Work out the finished part from the listing and answer in its coordinate system (mm). Face numbers are marked on the shaded views. A direction names the side the tool comes from. Round coordinates to 2 decimals unless told otherwise and drop trailing zeros. Order: outer loops, then holes, each group sorted by start corner. A loop starts at its lowest first (then second) coordinate and runs counter-clockwise, first axis right, second up. Notation, with made-up numbers: (37, -21.5) -> (85, -21.5) arc R21 cw to (85, 12.5) -> close; hole circle Ø9 at (69, 63.5). An arc over 180 degrees is marked (long way). Use one line per item in the form item = value.
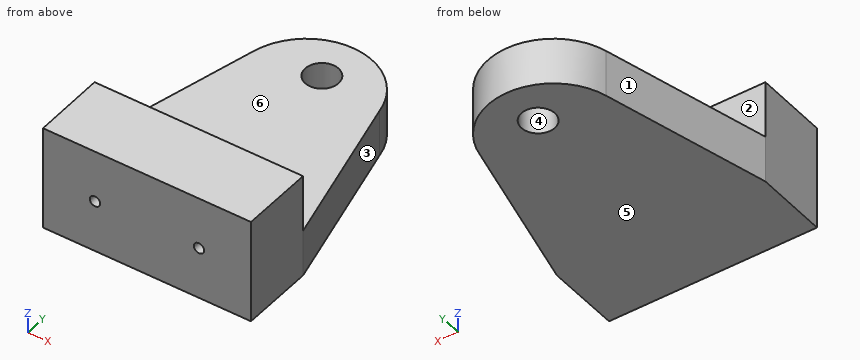
Autodesk Inventor part; units mm, degrees
ref_plane "YZ Plane" through (0, 0, 0) normal (1, 0, 0) x (0, 1, 0)
ref_plane "XZ Plane" through (0, 0, 0) normal (0, 1, 0) x (-1, 0, 0)
ref_plane "XY Plane" through (0, 0, 0) normal (0, 0, 1) x (1, 0, 0)
sketch "Sketch1" plane through (0, 0, 0) normal (0, 0, 1) x (1, 0, 0)
  circle A0 centre (10, 23.5) radius 1.6
  line L0 (-0.0511, 6.9998) -> (3.884, 22.9404)
  line L1 (20, 6.9998) -> (16.1838, 22.6325)
  arc A1 (16.1838, 22.6325) -> (3.884, 22.9404) centre (10, 21.4305) ccw
  line L2 (0, 0) -> (20, 0)
  line L3 (20, 6.9998) -> (16.1838, 22.6325)
  line L4 (0, 0) -> (-0.0511, 6.9998)
  line L5 (20, 0) -> (20, 6.9998)
  dimension "d17" = 7
  dimension "d18" = 6.9998
sketch "Sketch3" plane through (0, 0, 0) normal (0, 0, 1) x (1, 0, 0)
  point P0 (0, 0)
extrude "Extrusion1" add sketch "Sketch1" along normal blind 4.5
sketch "Sketch4" plane through (0, 0, 4.5) normal (0, 0, 1) x (1, 0, 0)
  line L0 (-0.0511, 6.9998) -> (0, 0)
  line L1 (20, 0) -> (20, 6.9998)
  line L2 (0, 0) -> (20, 0)
  line L3 (20, 0) -> (20, 6.9998)
  line L4 (3.884, 22.9404) -> (-0.0511, 6.9998)
  line L5 (20, 6.9998) -> (-0.0511, 6.9998)
  line L6 (0, 6.9998) -> (0, 0)
extrude "Extrusion2" add sketch "Sketch4" along normal blind 5.5
sketch "Sketch5" plane through (0, 0, 0) normal (0, -1, 0) x (1, 0, 0)
  circle A0 centre (5, 5) radius 0.5
  circle A1 centre (15, 5) radius 0.5
  point P0 (0, 0)
  dimension "d13" = 1
  dimension "d14" = 1
extrude "Extrusion3" cut sketch "Sketch5" against normal blind 5.5
properties part number "upper_deck_shaft_mount"
Item 1: The part is cut by section D-D, the plane z = 5. Give the vertices of the cut face in (x, y).
Findings:
outline = (-0.05, 7) -> (0, 0) -> (4.5, 0) -> (4.5, 5.5) -> (5.5, 5.5) -> (5.5, 0) -> (14.5, 0) -> (14.5, 5.5) -> (15.5, 5.5) -> (15.5, 0) -> (20, 0) -> (20, 7) -> close
Item 2: For the marked faces 5 and 6, determine the directions among +Z, -Z, +X, -X, +Y, -Y from which every point of the face is accessible in a straight line to the end or side of a thin tool.
Findings:
face_5 = -Z, +X, -X, +Y, -Y
face_6 = +Z, +X, -X, +Y
Item 3: Flat-ended cylindrical pins translate along their axes: P1, Ø0.8, axis at x = 15, z = 5, coming from the -Y side; P2, Ø1, axis at x = 15, z = 3, coming from the +Y side; P3, Ø6, axis at x = 12.5, y = 22, coming from the +Z side. Find the tip coordinate at first contact, or state that the pin passes through.
Findings:
P1 = 5.5
P2 = 25.84
P3 = 4.5
Item 4: The part is cut by section A-A, the plane x = 10. Give the vertices of the cut face in (y, z).
Findings:
outline = (0, 0) -> (21.9, 0) -> (21.9, 4.5) -> (7, 4.5) -> (7, 10) -> (0, 10) -> close; (25.1, 0) -> (27.73, 0) -> (27.73, 4.5) -> (25.1, 4.5) -> close
Item 5: The part is cut by section B-B, the plane z = 1. Give the vertices of the cut face in (x, y).
Findings:
outline = (-0.05, 7) -> (0, 0) -> (20, 0) -> (20, 7) -> (16.18, 22.63) arc R6.3 ccw to (3.88, 22.94) -> close; hole circle Ø3.2 at (10, 23.5)
Item 6: Determine the mould class of the marked faces 1, 2, 3 and 4 for opening direction X: released by +X, released by -X, zero draft, split by the parting line, or undercut.
Findings:
face_1 = released by -X
face_2 = zero draft
face_3 = released by +X
face_4 = undercut
Item 7: Consider line 1 along Z through (x, y) = (15, 3.4); line 2 along Y through (x, z) = (4.5, 7.75); line 3 along Z through (x, y) = (7.75, 23.25). Determine where each line is inside the solid, lowest interval first.
Findings:
line_1 = 0 to 4.5, 5.5 to 10
line_2 = 0 to 7
line_3 = 0 to 4.5
Item 8: The part is cut by section C-C, the plane y = 23.5. Give the vertices of the cut face in (x, z).
Findings:
outline = (4.05, 0) -> (8.4, 0) -> (8.4, 4.5) -> (4.05, 4.5) -> close; (11.6, 0) -> (15.95, 0) -> (15.95, 4.5) -> (11.6, 4.5) -> close
